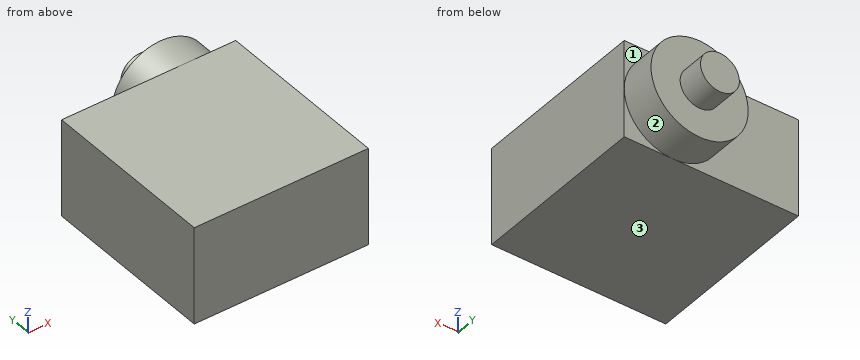
from build123d import *

# Parameters (mm, degrees)
BOSS_EXTRUDE2_DEPTH      = 11.4
BOSS_EXTRUDE2_DEPTH_BACK = 11.4
SKETCH1_W                = 22.4
SKETCH1_H                = 12.5
SKETCH3_R                = 6.25
BOSS_EXTRUDE3_DEPTH      = 4.6
SKETCH4_R                = 2.5
BOSS_EXTRUDE4_DEPTH      = 3.5


with BuildPart() as part:
    # Sketch1 → Boss-Extrude2 (new, two sides: drawn at the far end of the back side and taken through both)
    with BuildSketch(Plane(origin=(0, 0, 0), x_dir=(1, 0, 0), z_dir=(0, 1, 0)).offset(-BOSS_EXTRUDE2_DEPTH_BACK)):
        Rectangle(SKETCH1_W, SKETCH1_H)
    extrude(amount=BOSS_EXTRUDE2_DEPTH + BOSS_EXTRUDE2_DEPTH_BACK)

    # Sketch3 → Boss-Extrude3 (add)
    with BuildSketch(Plane(origin=(0, 11.4, 0), x_dir=(1, 0, 0), z_dir=(0, 1, 0))):
        with Locations(Location((4.95, 0, 0), (0, 0, 270))):
            Circle(SKETCH3_R)
    extrude(amount=BOSS_EXTRUDE3_DEPTH)

    # Sketch4 → Boss-Extrude4 (add)
    with BuildSketch(Plane(origin=(0, 16, 0), x_dir=(1, 0, 0), z_dir=(0, 1, 0))):
        with Locations(Location((4.95, 0, 0), (0, 0, 270))):
            Circle(SKETCH4_R)
    extrude(amount=BOSS_EXTRUDE4_DEPTH)


solid = part.part
The model under review builds one solid part; all positions refer to its coordinate system, in mm. Face numbers are marked on the shaded views. A direction names the side the tool comes from. Give positions to 0.01 mm unless a question says otherwise; leave off trailing zeros. Write each loop counter-clockwise with the first axis right and the second up, starting at its lowest first coordinate (ties: lowest second). Pieces come first, ordered by that corner, then holes.
1. Wall thickness on L1, parallel to Y at x = 1, z = 3; L2, parallel to Y at x = -7, z = 1.25; L3, parallel to Z at x = 1, y = 14: over which ranges is each line inside the solid? List them lowest first.
2. Tool access review of the marked faces 1, 2 and 3: name each direction out of +Z, -Z, +X, -X, +Y, -Y from which nothing blocks a thin tool from reaching the whole face with its end or side.
3. Add section C-C, the plane z = -3. Write out the cut boundary in (x, y).
4. Add section B-B, the plane x = 6.75. Write out the cut boundary in (y, z), plus the area to 3 significant figures.
5. Add section A-A, the plane z = -1.5. Write out the cut boundary in (x, y).
6. Add section D-D, the plane x = 0. Write out the cut boundary in (y, z), plus the area to 3 significant figures.
7. For P1, Ø3, axis at x = 7, z = -4.5, coming from the +Y side; P2, Ø6, axis at x = -5.5, z = 0, coming from the +Y side; P3, Ø6, axis at y = 15, z = 0.5, coming from the +X side, all flat-tipped, find the tip position at first contact; note any pin that passes through.
Worked answers:
1. L1: y = -11.4 to 16
1. L2: y = -11.4 to 11.4
1. L3: z = -4.84 to 4.84
2. face 1: +Z, +X, +Y
2. face 2: +Y
2. face 3: -Z, +X, -X, +Y, -Y
3. outline: (-11.2, -11.4) - (11.2, -11.4) - (11.2, 11.4) - (10.43, 11.4) - (10.43, 16) - (-0.53, 16) - (-0.53, 11.4) - (-11.2, 11.4) - close
4. outline: (-11.4, -6.25) - (11.4, -6.25) - (11.4, -5.99) - (16, -5.99) - (16, -1.73) - (19.5, -1.73) - (19.5, 1.73) - (16, 1.73) - (16, 5.99) - (11.4, 5.99) - (11.4, 6.25) - (-11.4, 6.25) - close
4. area: 352 mm2
5. outline: (-11.2, -11.4) - (11.2, -11.4) - (11.2, 11.4) - (11.02, 11.4) - (11.02, 16) - (6.95, 16) - (6.95, 19.5) - (2.95, 19.5) - (2.95, 16) - (-1.12, 16) - (-1.12, 11.4) - (-11.2, 11.4) - close
6. outline: (-11.4, -6.25) - (11.4, -6.25) - (11.4, -3.82) - (16, -3.82) - (16, 3.82) - (11.4, 3.82) - (11.4, 6.25) - (-11.4, 6.25) - close
6. area: 320 mm2
7. P1: stops at y = 16
7. P2: stops at y = 11.4
7. P3: stops at x = 11.2
